The figure shows three views and two pictorial views of one solid part (mm, origin at its lowest corner). Answer the questions. A direction names the side the tool comes from. Coordinates: 2 decimals unless noted, no trailing zeros. Order: outer loops, then holes, each group sorted by start corner. A loop starts at its lowest first (then second) coordinate and runs counter-clockwise, first axis right, second up. Notation, with made-up numbers: (32, 76) - (75, 76) arc R24 ccw to (75, 87) - close; hole circle Ø7 at (54, 61). An arc over 180 degrees is marked (long way). Use one line per item in the form item = value.
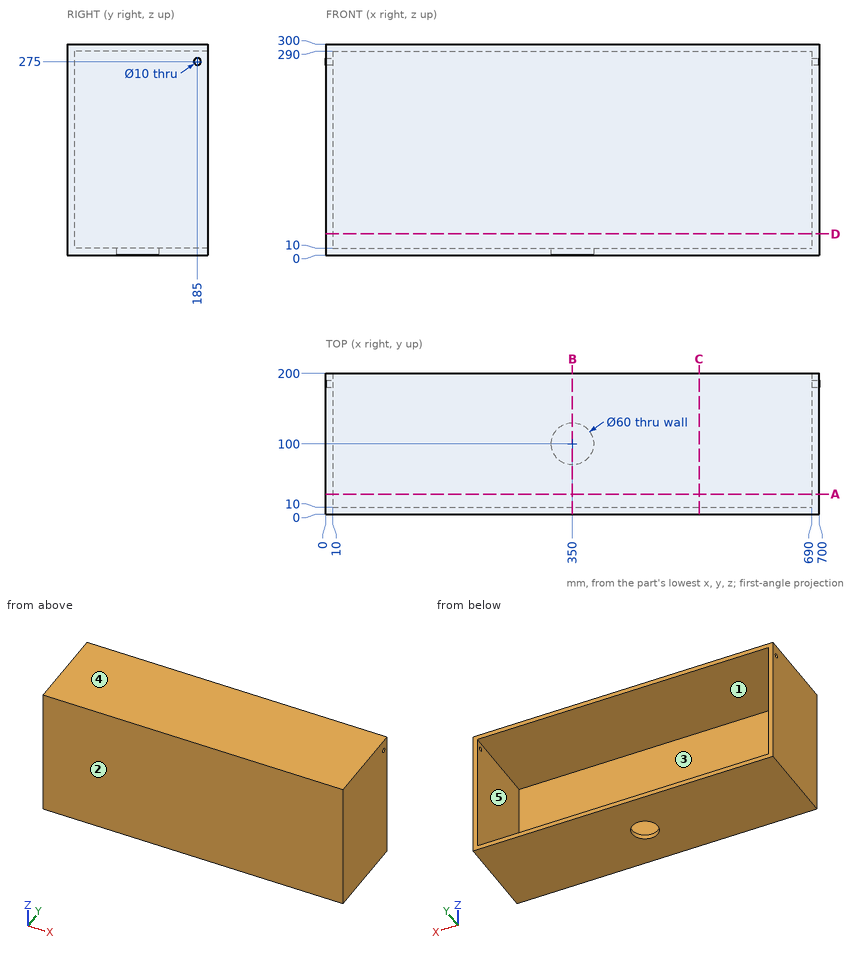
(1) Section C-C, the plane x = 530 is taken. Write down the section's boundary in (y, z), then the cut area to 3 significant figures.
Answer list:
outline = (0, 0) - (200, 0) - (200, 10) - (10, 10) - (10, 290) - (200, 290) - (200, 300) - (0, 300) - close
area = 6,800 mm2
(2) Section B-B, the plane x = 350 is taken. Write down the section's boundary in (y, z).
Answer list:
outline = (0, 0) - (70, 0) - (70, 10) - (10, 10) - (10, 290) - (200, 290) - (200, 300) - (0, 300) - close; (130, 0) - (200, 0) - (200, 10) - (130, 10) - close
(3) The mould has two halves that part along Y. Classify the marked faces 1, 2 and 3: +Y half, -Y half, draft (parallel to the pull), parting line (faces both ways), or undercut.
Answer list:
face_1 = draft
face_2 = -Y half
face_3 = +Y half
(4) Section D-D, the plane z = 30.5 is taken. Write down the section's boundary in (x, y), then the cut area to 3 significant figures.
Answer list:
outline = (0, 0) - (700, 0) - (700, 200) - (690, 200) - (690, 10) - (10, 10) - (10, 200) - (0, 200) - close
area = 10,800 mm2
(5) Which of the six approach directions +Z, -Z, +X, -X, +Y, -Y give full straight-line access (tool end or side, diameter ignored) to the marked faces 4 and 5?
Answer list:
face_4 = +Z, +X, -X, +Y, -Y
face_5 = +Y
(6) Given pin 1 Ø6 at (y, z) = (185, 275) entering from +X, flat-ended and moving along its own axis, determine where the tip first touches the part or whether it passes through.
Answer list:
pin_1 = through
(7) Straight lines are drawn through the part: L1, parallel to Y at x = 5, z = 275; L2, parallel to X at y = 161.5, z = 110; L3, parallel to Y at x = 350, z = 4. For each, find the intervals that lie inside material, in ascending order.
Answer list:
L1 = 0 to 180, 190 to 200
L2 = 0 to 10, 690 to 700
L3 = 0 to 70, 130 to 200
(8) Section A-A, the plane y = 28.5 is taken. Write down the section's boundary in (x, z).
Answer list:
outline = (0, 0) - (700, 0) - (700, 300) - (0, 300) - close; hole (10, 10) - (690, 10) - (690, 290) - (10, 290) - close
